Read the model definition and answer for the solid it produces. Units are mm, in the model's axes. Face numbers are marked on the shaded views. A direction names the side the tool comes from. Coordinates: 2 decimals unless noted, no trailing zeros. Loops run counter-clockwise (first coordinate to the right, second up) from the corner with the lowest first, then second, coordinate; pieces in that order, holes last.
from build123d import *

# Parameters (mm, degrees)
SKETCH1_W           = 105.1
SKETCH1_H           = 115
BOSS_EXTRUDE1_DEPTH = 10
BOSS_EXTRUDE2_DEPTH = 115
SKETCH2_R           = 2
CUT_EXTRUDE1_DEPTH  = 20
SKETCH4_R           = 4.25
CUT_EXTRUDE2_DEPTH  = 40


with BuildPart() as part:
    # Sketch1 → Boss-Extrude1 (new body)
    with BuildSketch(Plane(origin=(0, 0, 0), x_dir=(1, 0, 0), z_dir=(0, 1, 0))):
        Rectangle(SKETCH1_W, SKETCH1_H)
    extrude(amount=BOSS_EXTRUDE1_DEPTH)

    # Sketch3 → Boss-Extrude2 (add)
    with BuildSketch(Plane.XY.offset(57.5)):
        Polygon((-34.95, 10), (52.55, 10), (-34.95, 22.5), align=None)
    extrude(amount=-BOSS_EXTRUDE2_DEPTH)

    # Sketch2 → Cut-Extrude1 (cut)
    with BuildSketch(Plane.XZ):
        with Locations(Location((22.55, 23, 0), (0, 0, 270))):
            Circle(SKETCH2_R)
        with Locations(Location((2.631415713, 11.5, 0), (0, 0, 270))):
            Circle(SKETCH2_R)
        with Locations(Location((2.631415713, -11.5, 0), (0, 0, 270))):
            Circle(SKETCH2_R)
        with Locations(Location((22.55, -23, 0), (0, 0, 270))):
            Circle(SKETCH2_R)
        with Locations(Location((42.468584287, -11.5, 0), (0, 0, 270))):
            Circle(SKETCH2_R)
        with Locations(Location((42.468584287, 11.5, 0), (0, 0, 270))):
            Circle(SKETCH2_R)
    extrude(amount=-CUT_EXTRUDE1_DEPTH, mode=Mode.SUBTRACT)

    # Sketch4 → Cut-Extrude2 (cut)
    with BuildSketch(Plane(origin=(0, 50, 0), x_dir=(-1, 0, 0), z_dir=(0, -1, 0))):
        with Locations((-22.55, 23)):
            Circle(SKETCH4_R)
        with Locations((-2.631415713, 11.5)):
            Circle(SKETCH4_R)
        with Locations((-2.631415713, -11.5)):
            Circle(SKETCH4_R)
        with Locations((-22.55, -23)):
            Circle(SKETCH4_R)
        with Locations((-42.468584287, -11.5)):
            Circle(SKETCH4_R)
        with Locations((-42.468584287, 11.5)):
            Circle(SKETCH4_R)
    extrude(amount=CUT_EXTRUDE2_DEPTH, mode=Mode.SUBTRACT)


solid = part.part
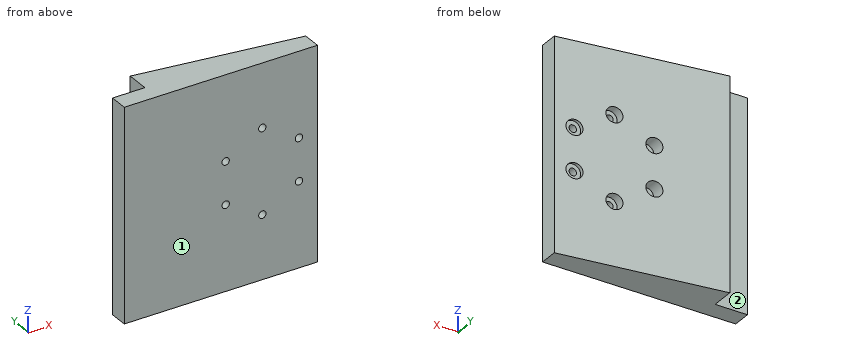
Item 1: A cutting plane is placed at B-B on x = 22.55. Determine the outline of the cut face in (y, z).
Numbers:
outline: (0, -57.5) - (14.29, -57.5) - (14.29, -27.25) - (10, -27.25) - (10, -25) - (0, -25) - close; (0, -21) - (10, -21) - (10, -18.75) - (14.29, -18.75) - (14.29, 18.75) - (10, 18.75) - (10, 21) - (0, 21) - close; (0, 25) - (10, 25) - (10, 27.25) - (14.29, 27.25) - (14.29, 57.5) - (0, 57.5) - close
Item 2: Find the intervals of material crossed by line 1 along X through (y, z) = (2.75, 11.5); line 2 along X through (y, z) = (3.75, -23), in increasing order.
Numbers:
line 1: x = -52.55 to 0.63, 4.63 to 40.47, 44.47 to 52.55
line 2: x = -52.55 to 20.55, 24.55 to 52.55
Item 3: A cutting plane is placed at D-D on z = 38. Determine the outline of the cut face in (x, y), then the cut area to 3 significant figures.
Numbers:
outline: (-52.55, 0) - (52.55, 0) - (52.55, 10) - (-34.95, 22.5) - (-34.95, 10) - (-52.55, 10) - close
area: 1,600 mm2
Item 4: A cutting plane is placed at C-C on z = 11.5. Determine the outline of the cut face in (x, y).
Numbers:
outline: (-52.55, 0) - (0.63, 0) - (0.63, 10) - (-1.62, 10) - (-1.62, 17.74) - (-34.95, 22.5) - (-34.95, 10) - (-52.55, 10) - close; (4.63, 0) - (40.47, 0) - (40.47, 10) - (38.22, 10) - (38.22, 12.05) - (6.88, 16.52) - (6.88, 10) - (4.63, 10) - close; (44.47, 0) - (52.55, 0) - (52.55, 10) - (46.72, 10.83) - (46.72, 10) - (44.47, 10) - close
Item 5: Which of the six approach directions +Z, -Z, +X, -X, +Y, -Y give full straight-line access (tool end or side, diameter ignored) to the marked faces 1 and 2?
Numbers:
face 1: +Z, -Z, +X, -X, -Y
face 2: +Z, -Z, -X, +Y
Item 6: Given pin 1 (2.5 mm diameter, centred on x = 42.5, z = -13.5, fed in from +Y); pin 2 (5 mm diameter, centred on x = 26.5, z = 7.5, fed in from +Y); pin 3 (9.5 mm diameter, centred on x = 22, z = 23, fed in from +Y), each flat-ended and moving along its own axis, determine where each tip first touches the part or whether it passes through.
Numbers:
pin 1: stops at y = 10
pin 2: stops at y = 14.08
pin 3: stops at y = 15.04
Item 7: A cutting plane is placed at A-A on z = 23. Determine the outline of the cut face in (x, y), then the cut area to 3 significant figures.
Numbers:
outline: (-52.55, 0) - (20.55, 0) - (20.55, 10) - (18.3, 10) - (18.3, 14.89) - (-34.95, 22.5) - (-34.95, 10) - (-52.55, 10) - close; (24.55, 0) - (52.55, 0) - (52.55, 10) - (26.8, 13.68) - (26.8, 10) - (24.55, 10) - close
area: 1,520 mm2
